Geometry check sheet. Reference: the model listing, model coordinates, mm. Face numbers are marked on the shaded views. A direction names the side the tool comes from. Give positions to 0.01 mm unless a question says otherwise; leave off trailing zeros. Write each loop counter-clockwise with the first axis right and the second up, starting at its lowest first coordinate (ties: lowest second). Pieces come first, ordered by that corner, then holes. Notation, with made-up numbers: (-19.75, -23) -> (-8.75, -23) arc R24 ccw to (-8.75, 3) -> close; hole circle Ø9 at (39, -31). An arc over 180 degrees is marked (long way). One line per item, written item: value.
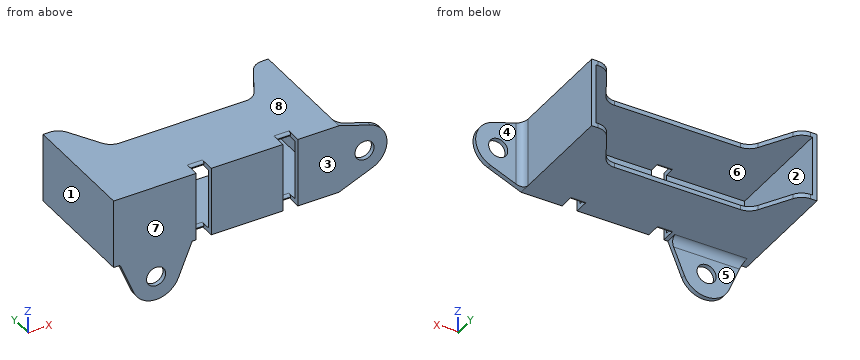
from build123d import *

# Parameters (mm, degrees)
SKETCH15_W                  = 75
SKETCH15_H                  = 23
SKETCH15_W_2                = 72
SKETCH15_H_2                = 20
BOSS_EXTRUDE8_DEPTH         = 38
BOSS_EXTRUDE11_DEPTH        = 1.5
F_1_4_0_25_DIAMETER_HOLE1_D = 6.35
SKETCH21_W                  = 5
SKETCH21_H                  = 4
CUT_EXTRUDE1_DEPTH          = 70.535961919
FILLET1_R                   = 5
FILLET2_R                   = 1
FILLET3_R                   = 2.5


with BuildPart() as part:
    # Sketch15 → Boss-Extrude8 (new body)
    with BuildSketch(Plane(origin=(0, 0, 0), x_dir=(1, 0, 0), z_dir=(0, 1, 0))):
        Rectangle(SKETCH15_W, SKETCH15_H)
        Rectangle(SKETCH15_W_2, SKETCH15_H_2, mode=Mode.SUBTRACT)
    extrude(amount=BOSS_EXTRUDE8_DEPTH)

    # Sketch18 → Boss-Extrude11 (add)
    with BuildSketch(Plane.XZ):
        with BuildLine():
            Line((-37.5, 11.5), (37.5, 11.5))
            Line((37.5, 11.5), (47.964864865, 8.110810811))
            ThreePointArc((47.964864865, 8.110810811), (53.493344425, 0.826258956), (48.576923077, -6.884615385))
            Line((48.576923077, -6.884615385), (37.5, -11.5))
            Line((37.5, -11.5), (-11.354744065, -11.5))
            Line((-11.354744065, -11.5), (-15.970166575, -22.576940483))
            ThreePointArc((-15.970166575, -22.576940483), (-23.354774707, -27.5), (-30.739382839, -22.576940483))
            Line((-30.739382839, -22.576940483), (-35.35480535, -11.5))
            Line((-35.35480535, -11.5), (-37.5, -11.5))
            Line((-37.5, -11.5), (-37.5, 11.5))
        make_face()
    extrude(amount=BOSS_EXTRUDE11_DEPTH)

    # 1/4 (0.25) Diameter Hole1 (through all)
    with Locations(Plane(origin=(0, 0, 0), x_dir=(1, 0, 0), z_dir=(0, 1, 0))):
        with Locations((46, 0), (-23.354774707, 19.5)):
            Hole(F_1_4_0_25_DIAMETER_HOLE1_D / 2)

    # Sketch21 → Cut-Extrude1 (cut, through all)
    with BuildSketch(Plane(origin=(0, 0, -11.5), x_dir=(-1, 0, 0), z_dir=(0, 0, -1))):
        Polygon((-32.5, 38), (-23.839745962, 23), (23.839745962, 23), (32.5, 38), align=None)
        with Locations((-21.339745962, 0.5)):
            Rectangle(SKETCH21_W, SKETCH21_H)
        with Locations((7.5, 0.5)):
            Rectangle(SKETCH21_W, SKETCH21_H)
    extrude(amount=-CUT_EXTRUDE1_DEPTH, mode=Mode.SUBTRACT)

    # Fillet1
    fillet1_edges = [part.edges().sort_by_distance(p)[0] for p in [
        (32.5, 38, -10.75),
        (-32.5, 38, -10.75),
        (-23.839745962, 23, -10.75),
        (23.839745962, 23, -10.75),
        (32.5, 38, 10.75),
        (-32.5, 38, 10.75),
        (-23.839745962, 23, 10.75),
        (23.839745962, 23, 10.75),
    ]]
    fillet(fillet1_edges, radius=FILLET1_R)

    # Fillet2
    # the kernel refuses this fillet: 1 mm, written as the material it takes off along each edge
    with BuildSketch(Plane(origin=(18.839745962, 2.5, -11.5), x_dir=(0, 1, 0), z_dir=(1, 0, 0)), Plane(origin=(23.839745962, 2.5, -10), x_dir=(0, 1, 0), z_dir=(-1, 0, 0)), Plane(origin=(18.839745962, 2.5, 10), x_dir=(0, 1, 0), z_dir=(1, 0, 0)), Plane(origin=(23.839745962, 2.5, 11.5), x_dir=(0, 1, 0), z_dir=(-1, 0, 0)), Plane(origin=(-10, 2.5, -11.5), x_dir=(0, 1, 0), z_dir=(1, 0, 0)), Plane(origin=(-5, 2.5, -10), x_dir=(0, 1, 0), z_dir=(-1, 0, 0)), Plane(origin=(-10, 2.5, 10), x_dir=(0, 1, 0), z_dir=(1, 0, 0)), Plane(origin=(-5, 2.5, 11.5), x_dir=(0, 1, 0), z_dir=(-1, 0, 0))) as fillet2_piece_1:
        with BuildLine():
            CenterArc((FILLET2_R, FILLET2_R), FILLET2_R, 180, 90)
            Line((0, FILLET2_R), (0, 0))
            Line((0, 0), (FILLET2_R, 0))
        make_face()
    extrude(amount=5, mode=Mode.SUBTRACT)

    # Fillet3
    fillet3_edges = [part.edges().sort_by_distance(p)[0] for p in [
        (-23.354774707, 0, -11.5),
        (37.5, 0, 0),
    ]]
    fillet(fillet3_edges, radius=FILLET3_R)


solid = part.part
1) Scan lines: probe 1 along X at (y, z) = (18.5, -1.5); probe 2 along Z at (x, y) = (-6, 14); probe 3 along Y at (x, z) = (-3, 3). Record each from-to range of solid material in increasing order.
Verdict:
probe 1: -37.5 to -36, 36 to 37.5
probe 2: -11.5 to -10, 10 to 11.5
probe 3: -1.5 to 0
2) Mould release check, pull along X, two halves, no side actions. Record for the marked faces 1, 2 and 3: released by +X, released by -X, zero draft, split by the parting line, or undercut.
Verdict:
face 1: released by -X
face 2: undercut
face 3: zero draft
3) Sectioned sample at B-B on z = -5.5. Record the cut outline in (x, y).
Verdict:
outline: (-37.5, -1.5) -> (-10, -1.5) -> (-10, 0) -> (-36, 0) -> (-36, 38) -> (-37.5, 38) -> close; (-5, -1.5) -> (18.84, -1.5) -> (18.84, 0) -> (-5, 0) -> close; (23.84, -1.5) -> (50.79, -1.5) -> (50.79, 0) -> (40, 0) arc R2.5 cw to (37.5, 2.5) -> (37.5, 38) -> (36, 38) -> (36, 0) -> (23.84, 0) -> close
4) Sectioned sample at D-D on z = -21.5. Record the cut outline in (x, y).
Verdict:
outline: (-31.19, -1.5) -> (-25.82, -1.5) -> (-25.82, 0) -> (-31.19, 0) -> close; (-20.89, -1.5) -> (-15.52, -1.5) -> (-15.52, 0) -> (-20.89, 0) -> close
5) Sectioned sample at C-C on x = 15.5. Record the cut outline in (y, z).
Verdict:
outline: (-1.5, -11.5) -> (23, -11.5) -> (23, -10) -> (0, -10) -> (0, 10) -> (23, 10) -> (23, 11.5) -> (-1.5, 11.5) -> close
6) Depth check by flat-ended pin: pin 1 Ø7.5 at (x, z) = (-23.35, -19.5) entering from +Y; pin 2 Ø8 at (x, z) = (4.5, -17.5) entering from +Y; pin 3 Ø0.8 at (x, z) = (-4.5, -11) entering from +Y; pin 4 Ø1 at (y, z) = (11, -1.5) entering from +X. Enter the tip coordinate at first touch or a pass-through.
Verdict:
pin 1: y = 0
pin 2: through
pin 3: y = 23
pin 4: x = 37.5
7) Sectioned sample at A-A on y = 18. Record the cut outline in (x, z), plus the area to 3 significant figures.
Verdict:
outline: (-37.5, -11.5) -> (37.5, -11.5) -> (37.5, 11.5) -> (-37.5, 11.5) -> close; hole (-36, -10) -> (36, -10) -> (36, 10) -> (-36, 10) -> close
area: 285 mm^2
8) Tool access check on the marked faces 4, 5, 6, 7 and 8. Record the directions out of +Z, -Z, +X, -X, +Y, -Y that give a thin tool (end or side, any length) a straight path to the whole face; none if there is none.
Verdict:
face 4: +Z, -Z, +X, +Y
face 5: -Z, +X, -X, +Y
face 6: +Y
face 7: +Z, -Z, +X, -X, -Y
face 8: +Z, +X, -X, +Y, -Y
